from build123d import *

# Parameters (mm, degrees)
F0_W     = 76
F0_H     = 76
F0_W_2   = 68
F0_H_2   = 68
F1_DEPTH = 4
F2_DEPTH = 19
F3_R     = 6
F4_R     = 10
F5_R     = 1.2


with BuildPart() as f1:
    # F0 (on Top) → F1 (new body)
    with BuildSketch(Plane.XY):
        Rectangle(F0_W, F0_H)
        Rectangle(F0_W_2, F0_H_2, mode=Mode.SUBTRACT)
        Rectangle(F0_W_2, F0_H_2)
    extrude(amount=F1_DEPTH)

    # F0 (on Top) → F2 (join)
    with BuildSketch(Plane.XY):
        Rectangle(F0_W, F0_H)
        Rectangle(F0_W_2, F0_H_2, mode=Mode.SUBTRACT)
    extrude(amount=F2_DEPTH)

    # F3
    f3_edges = [f1.edges().sort_by_distance(p)[0] for p in [
        (34, 34, 11.5),
        (34, -34, 11.5),
        (-34, -34, 11.5),
        (-34, 34, 11.5),
    ]]
    fillet(f3_edges, radius=F3_R)

    # F4
    f4_edges = [f1.edges().sort_by_distance(p)[0] for p in [
        (-38, -38, 9.5),
        (38, -38, 9.5),
        (38, 38, 9.5),
        (-38, 38, 9.5),
    ]]
    fillet(f4_edges, radius=F4_R)

    # F5
    f5_edges = [f1.edges().sort_by_distance(p)[0] for p in [
        (34, 0, 4),
    ]]
    fillet(f5_edges, radius=F5_R)


solid = f1.part
Part model, mm, in its own coordinate system. A direction names the side the tool comes from. Give positions to 0.01 mm unless a question says otherwise; leave off trailing zeros. Write each loop counter-clockwise with the first axis right and the second up, starting at its lowest first coordinate (ties: lowest second). Pieces come first, ordered by that corner, then holes.
1) Cut at B-B on y = -18. Write the cut outline in (x, z), then the cut area to 3 significant figures.
Resolved:
outline: (-38, 0) - (38, 0) - (38, 19) - (34, 19) - (34, 5.2) arc R1.2 cw to (32.8, 4) - (-32.8, 4) arc R1.2 cw to (-34, 5.2) - (-34, 19) - (-38, 19) - close
area: 425 mm2
2) Which spindle directions (+Z, -Z, +X, -X, +Y, -Y) get a long thin tool onto all of the face, cutting with end or side? Do faces 1 (the face through (32.289, -32.196, 12.197)), 2 (the face through (38, 0, 9)). Say none if no direction does.
Resolved:
face 1: +Z
face 2: +Z, -Z, +X, +Y, -Y
3) Pin check, flat tip, straight feed: pin 1 (19.5 mm diameter, centred on x = 1, y = -12.5, fed in from +Z). Stop position of the tip, or through.
Resolved:
pin 1: stops at z = 4
4) Probe L1, parallel to Y at x = 25, z = 11.25; L2, parallel to Z at x = -8.5, y = 8. List the from-to ranges inside material, lowest first.
Resolved:
L1: y = -38 to -34, 34 to 38
L2: z = 0 to 4
5) Two-plate mould, pull along Y, no slides. Class faces 3 (the face through (-3, -36, 19)), 4 (the face through (34.99, 35.15, 9.37)), 5 (the face through (-32.289, -32.196, 12.197)): released by +Y, released by -Y, zero draft, split by the parting line, or undercut.
Resolved:
face 3: zero draft
face 4: released by +Y
face 5: undercut
6) Cut at A-A on z = 12. Write the cut outline in (x, y), then the cut area to 3 significant figures.
Resolved:
outline: (-38, -28) arc R10 ccw to (-28, -38) - (28, -38) arc R10 ccw to (38, -28) - (38, 28) arc R10 ccw to (28, 38) - (-28, 38) arc R10 ccw to (-38, 28) - close; hole (-34, -28) arc R6 ccw to (-28, -34) - (28, -34) arc R6 ccw to (34, -28) - (34, 28) arc R6 ccw to (28, 34) - (-28, 34) arc R6 ccw to (-34, 28) - close
area: 1,100 mm2
